```python
from build123d import *

# Parameters (mm, degrees)
F3_D           = 5
F3_CBORE_D     = 10
F3_CBORE_DEPTH = 5
F4_T6_ANGLE    = 291.5048547237
F4_T14_ANGLE   = 80.1015252238


# Not quite as in the source:
# - a fillet or chamfer that OpenCascade refuses, or shapes differently, is made with other operations: its cross-section is extruded or revolved along the edge and cut away or added


with BuildPart() as f1:
    # F0 (on Right) → F1 (revolve)
    with BuildSketch(Plane.YZ):
        Polygon((63.7261494994, 30.5484924465), (29.6720992774, 30.5484924465), (29.6720992774, -22.7861702442), (41.941575706, -22.7861702442), (41.941575706, -14.2726562917), (51.7070740461, -14.2726562917), (51.7070740461, -22.7861702442), (63.7261494994, -22.7861702442), align=None)
    revolve(axis=Axis((0, 0, 14.0182273462), (0, 0, 1)))

    # F3 (through all)
    with Locations(Plane.XY.offset(30.5484924465)):
        with Locations((10.9902555123, 46.0034860298), (49.8999916017, 14.0128545463)):
            CounterBoreHole(F3_D / 2, F3_CBORE_D / 2, F3_CBORE_DEPTH)

    # F4: chamfer of 3 on 7 edges, made by hand

    # F4_s1 → F4_t2 (revolve, cut)
    with BuildSketch(Plane.YZ):
        Polygon((60.7261494994, 30.5484924465), (63.7261494994, 27.5484924465), (63.7261494994, 30.5484924465), align=None)
    revolve(axis=Axis((0, 0, 30.5484924465), (0, 0, 1)), mode=Mode.SUBTRACT)

    # F4_s3 → F4_t4 (revolve, cut)
    with BuildSketch(Plane.YZ):
        Polygon((63.7261494994, -19.7861702442), (60.7261494994, -22.7861702442), (63.7261494994, -22.7861702442), align=None)
    revolve(axis=Axis((0, 0, -22.7861702442), (0, 0, 1)), mode=Mode.SUBTRACT)

    # F4_s5 → F4_t6 (revolve, cut)
    with BuildSketch(Plane.YZ):
        Polygon((54.7070740461, -22.7861702442), (51.7070740461, -19.7861702442), (51.7070740461, -22.7861702442), align=None)
    revolve(axis=Axis((0, 0, -22.7861702442), (0, 0, 1)), revolution_arc=F4_T6_ANGLE, mode=Mode.SUBTRACT)

    # F4_s7 → F4_t8 (revolve, cut)
    with BuildSketch(Plane.YZ):
        Polygon((38.941575706, -22.7861702442), (41.941575706, -19.7861702442), (41.941575706, -22.7861702442), align=None)
    revolve(axis=Axis((0, 0, -22.7861702442), (0, 0, 1)), mode=Mode.SUBTRACT)

    # F4_s9 → F4_t10 (revolve, cut)
    with BuildSketch(Plane.YZ):
        Polygon((29.6720992774, -19.7861702442), (32.6720992774, -22.7861702442), (29.6720992774, -22.7861702442), align=None)
    revolve(axis=Axis((0, 0, -22.7861702442), (0, 0, 1)), mode=Mode.SUBTRACT)

    # F4_s11 → F4_t12 (revolve, cut)
    with BuildSketch(Plane.YZ):
        Polygon((32.6720992774, 30.5484924465), (29.6720992774, 27.5484924465), (29.6720992774, 30.5484924465), align=None)
    revolve(axis=Axis((0, 0, 30.5484924465), (0, 0, 1)), mode=Mode.SUBTRACT)

    # F4_s13 → F4_t14 (revolve, cut)
    with BuildSketch(Plane(origin=(0, 0, 0), x_dir=(0, 0, 1), z_dir=(0.1719028764, -0.9851139026, 0))):
        Polygon((-22.7861702442, -54.7070740461), (-19.7861702442, -51.7070740461), (-22.7861702442, -51.7070740461), align=None)
    revolve(axis=Axis((0, 0, -22.7861702442), (0, 0, 1)), revolution_arc=F4_T14_ANGLE, mode=Mode.SUBTRACT)


solid = f1.part
```
The listing builds one solid part. Answer for the finished solid, in the listing's coordinates (mm). A direction names the side the tool comes from. Coordinates: 2 decimals unless noted, no trailing zeros. Write each loop counter-clockwise with the first axis right and the second up, starting at its lowest first coordinate (ties: lowest second). Pieces come first, ordered by that corner, then holes. Notation, with made-up numbers: (-26.5, 69.25) - (16.5, 69.25) arc R15 ccw to (16.5, 75.25) - close; hole circle Ø3 at (6, 73). An arc over 180 degrees is marked (long way). Return JSON: item names as keys, results as strings. Group by question number.
Q1. Find the intervals of material crossed by line 1 along X through (y, z) = (0, -16.35); line 2 along X through (y, z) = (0, 4.5); line 3 along X through (y, z) = (-26, -20), in increasing order. Write a range as [from, to].
Q2. The part is cut by section A-A on x = 0. Write down the section's boundary in (y, z).
Q3. The part is cut by section C-C on z = 17.5. Write down the section's boundary in (x, y), and give its area (3 significant figures).
Q4. For a pull along Y with two mould halves and no side action, classify faces 4 (the flat face through (-32, 9, -22.786)), 5 (the cylindrical face through (52.4, 14.1, 1.2)), 6 (the conical face through (-60.395, -7.93, 30.361)), 7 (the conical face through (29.109, -6.464, 27.694)) as +Y half, -Y half, draft (parallel to the pull), parting line (faces both ways), or undercut.
Q5. Which of the six approach directions +Z, -Z, +X, -X, +Y, -Y give full straight-line access (tool end or side, diameter ignored) to faces 1 (the cylindrical face through (44.905, 14.233, 28.083)), 2 (the flat face through (42, -4, -14.273)), 3 (the cylindrical face through (62.21, -13.81, 4.21))?
Q6. Flat-ended cylindrical pins translate along their axes: pin 1 Ø13 at (x, y) = (10.99, 46) entering from -Z; pin 2 Ø6 at (x, y) = (49.9, 14.01) entering from +Z; pin 3 Ø4 at (y, z) = (-16.5, 7) entering from +X. Find the tip coordinate at first contact, or state that the pin passes through.
Evaluation:
{
 "1": {"line 1": "x = [-63.73, -51.71], [-41.94, -29.67], [29.67, 41.94], [51.71, 63.73]", "line 2": "x = [-63.73, -29.67], [29.67, 63.73]", "line 3": "x = [-57.95, -44.94], [-32.64, -14.74], [14.74, 32.64], [44.94, 57.95]"},
 "2": {"outline": "(-63.73, -19.79) - (-60.73, -22.79) - (-54.71, -22.79) - (-51.71, -19.79) - (-51.71, -14.27) - (-41.94, -14.27) - (-41.94, -19.79) - (-38.94, -22.79) - (-32.67, -22.79) - (-29.67, -19.79) - (-29.67, 27.55) - (-32.67, 30.55) - (-60.73, 30.55) - (-63.73, 27.55) - close; (29.67, -19.79) - (32.67, -22.79) - (38.94, -22.79) - (41.94, -19.79) - (41.94, -14.27) - (51.71, -14.27) - (51.71, -19.79) - (54.71, -22.79) - (60.73, -22.79) - (63.73, -19.79) - (63.73, 27.55) - (60.73, 30.55) - (32.67, 30.55) - (29.67, 27.55) - close"},
 "3": {"outline": "circle Ø127.45 at (0, 0); hole circle Ø59.34 at (0, 0); hole circle Ø5 at (10.99, 46); hole circle Ø5 at (49.9, 14.01)", "area": "9,950 mm2"},
 "4": {"face 4": "draft", "face 5": "undercut", "face 6": "parting line", "face 7": "undercut"},
 "5": {"face 1": "+Z", "face 2": "-Z", "face 3": "+Z, -Z"},
 "6": {"pin 1": "stops at z = -21.87", "pin 2": "stops at z = 25.55", "pin 3": "stops at x = 62.05"}
}
